Design review of the part built by this model. Coordinates are the model's own, in mm. A direction names the side the tool comes from. Coordinates: 2 decimals unless noted, no trailing zeros. Write each loop counter-clockwise with the first axis right and the second up, starting at its lowest first coordinate (ties: lowest second). Pieces come first, ordered by that corner, then holes.
Q1. Take a section at B-B (y = 24). Give the boundary of the cut face in (x, z).
Q2. For probe 1 along Y at (x, z) = (-4.2, 0); probe 2 along X at (y, z) = (29.5, 0); probe 3 along X at (y, z) = (-38.75, 0), list the stretches that pass through material, from the lowest coordinate up.
Q3. Insertion check: pin 1 (2 mm diameter, centred on x = -1, y = 4.5, fed in from -Z); pin 2 (4 mm diameter, centred on y = -28.5, z = 1.5, fed in from -X); pin 3 (6 mm diameter, centred on x = 1.5, y = -12, fed in from -Z). Each pin has a flat end and moves straight along its axis. Give the tip position at first contact, or say it passes through.
Q4. Take a section at A-A (y = 10). Give the boundary of the cut face in (x, z).
Q5. Machinability: for faces 1 (the cylindrical face through (0.54, -43.45, -2.44)), 2 (the flat face through (2, -52.066, -2)), 3 (the flat face through (0, 14.934, 0)), 4 (the cylindrical face through (-5.27, 4.49, -1.17)), 5 (the cylindrical face through (-3.8, 23.98, -2.31)), which of the approach directions +Z, -Z, +X, -X, +Y, -Y give a long, thin tool a straight path to every point of the face, cutting with its end or side? Answer none if there is none.
Q6. Mouldability with a two-part tool opening along Z and no side actions: class faces 6 (the cylindrical face through (5.857, 21.972, -1.301)), 7 (the flat face through (-4, 2.934, 4)), 8 (the cylindrical face through (2.93, 27.26, -0.65)) as pulls with the +Z half, pulls with the -Z half, needs draft (parallel to the pull), parting line crosses it, or undercut.
```python
from build123d import *

# Parameters (mm, degrees)
CHAMFER1_SIZE         = 0.5
BOSS_EXTRUDE1_START   = -1.2
SKETCH2_R             = 7.5
SKETCH2_R_2           = 3
BOSS_EXTRUDE1_DEPTH   = 1.2
SKETCH5_R             = 2.5
CUT_EXTRUDE1_DEPTH    = 54.135491794
M6_TAPPED_HOLE1_D     = 5
M6_TAPPED_HOLE1_DEPTH = 17
M6_TAPPED_HOLE1_TIP   = 1.502151548


with BuildPart() as part:
    # Sketch1 → Revolve1 (revolve)
    with BuildSketch(Plane.XY, mode=Mode.PRIVATE) as revolve1_sk:
        Polygon((-3, 39.933883493), (-3, 14.933883493), (0, 14.933883493), (0, -52.066116507), (-5, -52.066116507), (-5, 2.933883493), (-6, 2.933883493), (-6, 39.933883493), align=None)
    revolve(revolve1_sk.sketch.rotate(Axis((0, 54.453238627, 0), (0, -1, 0)), 270), axis=Axis((0, 54.453238627, 0), (0, -1, 0)))

    # Chamfer1
    chamfer1_edges = [part.edges().sort_by_distance(p)[0] for p in [
        (0, -52.066116507, -5),
    ]]
    chamfer(chamfer1_edges, length=CHAMFER1_SIZE)

    # Sketch2 → Boss-Extrude1 (add)
    with BuildSketch(Plane(origin=(0, 39.933883493, 0), x_dir=(1, 0, 0), z_dir=(0, 1, 0)).offset(BOSS_EXTRUDE1_START)):
        with Locations(Location((0, 0, 0), (0, 0, 270))):
            Circle(SKETCH2_R)
        with Locations(Location((0, 0, 0), (0, 0, 270))):
            Circle(SKETCH2_R_2, mode=Mode.SUBTRACT)
    extrude(amount=BOSS_EXTRUDE1_DEPTH)

    # Sketch4 → Groove for ANSI B27.7 - 3BM1-12, Basic Internal Retaining Ring1 (revolve, cut)
    with BuildSketch(Plane(origin=(0, 54.453238627, 0), x_dir=(0, 0, 1), z_dir=(-1, 0, 0))):
        with BuildLine():
            Line((6.225, -50.219355134), (5.4, -50.219355134))
            Line((5.4, -50.219355134), (5.4, -49.719355134))
            Line((5.4, -49.719355134), (6.225, -49.719355134))
            ThreePointArc((6.225, -49.719355134), (6.295710678, -49.748644456), (6.325, -49.819355134))
            Line((6.325, -49.819355134), (6.325, -50.119355134))
            ThreePointArc((6.325, -50.119355134), (6.295710678, -50.190065812), (6.225, -50.219355134))
        make_face()
    revolve(axis=Axis((0, 4.453238627, 0), (0, 1, 0)), mode=Mode.SUBTRACT)

    # Sketch5 → Cut-Extrude1 (cut, through all)
    with BuildSketch(Plane(origin=(0, 0, 0), x_dir=(0, 0, -1), z_dir=(1, 0, 0))):
        with Locations((0, 24.933883493)):
            Circle(SKETCH5_R)
    extrude(amount=-CUT_EXTRUDE1_DEPTH, mode=Mode.SUBTRACT)

    # M6 Tapped Hole1
    with Locations(Plane.XZ.offset(52.066116507)):
        with Locations((0, 0)):
            Hole(M6_TAPPED_HOLE1_D / 2, depth=M6_TAPPED_HOLE1_DEPTH)
            with Locations((0, 0, -(M6_TAPPED_HOLE1_DEPTH + M6_TAPPED_HOLE1_TIP / 2))):  # 118° drill point
                Cone(0, M6_TAPPED_HOLE1_D / 2, M6_TAPPED_HOLE1_TIP, mode=Mode.SUBTRACT)


solid = part.part
```
Response:
1. outline: (-5.53, -2.32) arc R6 ccw (long way) to (-5.53, 2.32) - (-1.9, 2.32) arc R3 cw (long way) to (-1.9, -2.32) - close
2. probe 1: y = -52.07 to 22.43, 27.43 to 39.93
2. probe 2: x = -6 to -3, 3 to 6
2. probe 3: x = -5 to -2.5, 2.5 to 5
3. pin 1: stops at z = -6
3. pin 2: stops at x = -5
3. pin 3: stops at z = -5
4. outline: circle Ø12 at (0, 0)
5. face 1: -Y
5. face 2: +Z, -Z, +X, -X, -Y
5. face 3: +Y
5. face 4: none
5. face 5: -X
6. face 6: parting line crosses it
6. face 7: needs draft
6. face 8: undercut
